```python
from build123d import *

# Parameters (mm, degrees)
F1_DEPTH = 5
F2_R     = 27
F2_R_2   = 25.5
F3_DEPTH = 5


# Not quite as in the source:
# - a feature names something its author has since deleted; it is built from what else it names


with BuildPart() as f1:
    # F0 (on Top) → F1 (new body)
    with BuildSketch(Plane.XY):
        with BuildLine():
            Line((26.83281573, 3), (23.8117617996, 3))
            ThreePointArc((23.8117617996, 3), (23.9528942217, 1.502949901), (24, 0))
            ThreePointArc((24, 0), (23.9528942217, -1.502949901), (23.8117617996, -3))
            Line((23.8117617996, -3), (26.83281573, -3))
            ThreePointArc((26.83281573, -3), (26.9581715321, -1.5023274094), (27, 0))
            ThreePointArc((27, 0), (26.9581715321, 1.5023274094), (26.83281573, 3))
        make_face()
        with BuildLine():
            ThreePointArc((3, 23.8117617996), (16.9705627485, 16.9705627485), (23.8117617996, 3))
            Line((23.8117617996, 3), (26.83281573, 3))
            ThreePointArc((26.83281573, 3), (19.091883092, 19.091883092), (3, 26.83281573))
            Line((3, 26.83281573), (3, 23.8117617996))
        make_face()
        with BuildLine():
            Line((26.83281573, -3), (23.8117617996, -3))
            ThreePointArc((23.8117617996, -3), (16.9705627485, -16.9705627485), (3, -23.8117617996))
            Line((3, -23.8117617996), (3, -26.83281573))
            ThreePointArc((3, -26.83281573), (19.091883092, -19.091883092), (26.83281573, -3))
        make_face()
        with BuildLine():
            ThreePointArc((-3, 23.8117617996), (0, 24), (3, 23.8117617996))
            Line((3, 23.8117617996), (3, 26.83281573))
            ThreePointArc((3, 26.83281573), (0, 27), (-3, 26.83281573))
            Line((-3, 26.83281573), (-3, 23.8117617996))
        make_face()
        with BuildLine():
            ThreePointArc((-23.8117617996, 3), (-16.9705627485, 16.9705627485), (-3, 23.8117617996))
            Line((-3, 23.8117617996), (-3, 26.83281573))
            ThreePointArc((-3, 26.83281573), (-19.091883092, 19.091883092), (-26.83281573, 3))
            Line((-26.83281573, 3), (-23.8117617996, 3))
        make_face()
        with BuildLine():
            Line((-3, -26.83281573), (-3, -23.8117617996))
            ThreePointArc((-3, -23.8117617996), (-16.9705627485, -16.9705627485), (-23.8117617996, -3))
            Line((-23.8117617996, -3), (-26.83281573, -3))
            ThreePointArc((-26.83281573, -3), (-19.091883092, -19.091883092), (-3, -26.83281573))
        make_face()
        with BuildLine():
            ThreePointArc((3, -23.8117617996), (0, -24), (-3, -23.8117617996))
            Line((-3, -23.8117617996), (-3, -26.83281573))
            ThreePointArc((-3, -26.83281573), (0, -27), (3, -26.83281573))
            Line((3, -26.83281573), (3, -23.8117617996))
        make_face()
        with BuildLine():
            ThreePointArc((-23.8117617996, -3), (-24, 0), (-23.8117617996, 3))
            Line((-23.8117617996, 3), (-26.83281573, 3))
            ThreePointArc((-26.83281573, 3), (-27, 0), (-26.83281573, -3))
            Line((-26.83281573, -3), (-23.8117617996, -3))
        make_face()
        with BuildLine():
            ThreePointArc((-6.7372564891, -3), (-7.2138024511, -1.5335185674), (-7.375, 0))
            ThreePointArc((-7.375, 0), (-7.2138024511, 1.5335185674), (-6.7372564891, 3))
            Line((-6.7372564891, 3), (-23.8117617996, 3))
            ThreePointArc((-23.8117617996, 3), (-24, 0), (-23.8117617996, -3))
            Line((-23.8117617996, -3), (-6.7372564891, -3))
        make_face()
        with BuildLine():
            ThreePointArc((-4.875, 0), (-3.4471455583, 3.4471455583), (0, 4.875))
            Line((0, 4.875), (0, 7.375))
            ThreePointArc((0, 7.375), (-1.5335185674, 7.2138024511), (-3, 6.7372564891))
            ThreePointArc((-3, 6.7372564891), (-5.2149125113, 5.2149125113), (-6.7372564891, 3))
            ThreePointArc((-6.7372564891, 3), (-7.2138024511, 1.5335185674), (-7.375, 0))
            Line((-7.375, 0), (-4.875, 0))
        make_face()
        with BuildLine():
            Line((0, -7.375), (0, -4.875))
            ThreePointArc((0, -4.875), (-3.4471455583, -3.4471455583), (-4.875, 0))
            Line((-4.875, 0), (-7.375, 0))
            ThreePointArc((-7.375, 0), (-7.2138024511, -1.5335185674), (-6.7372564891, -3))
            ThreePointArc((-6.7372564891, -3), (-5.2149125113, -5.2149125113), (-3, -6.7372564891))
            ThreePointArc((-3, -6.7372564891), (-1.5335185674, -7.2138024511), (0, -7.375))
        make_face()
        with BuildLine():
            Line((7.375, 0), (4.875, 0))
            ThreePointArc((4.875, 0), (3.4471455583, -3.4471455583), (0, -4.875))
            Line((0, -4.875), (0, -7.375))
            ThreePointArc((0, -7.375), (1.5335185674, -7.2138024511), (3, -6.7372564891))
            ThreePointArc((3, -6.7372564891), (5.2149125113, -5.2149125113), (6.7372564891, -3))
            ThreePointArc((6.7372564891, -3), (7.2138024511, -1.5335185674), (7.375, 0))
        make_face()
        with BuildLine():
            ThreePointArc((0, 4.875), (3.4471455583, 3.4471455583), (4.875, 0))
            Line((4.875, 0), (7.375, 0))
            ThreePointArc((7.375, 0), (7.2138024511, 1.5335185674), (6.7372564891, 3))
            ThreePointArc((6.7372564891, 3), (5.2149125113, 5.2149125113), (3, 6.7372564891))
            ThreePointArc((3, 6.7372564891), (1.5335185674, 7.2138024511), (0, 7.375))
            Line((0, 7.375), (0, 4.875))
        make_face()
        with BuildLine():
            ThreePointArc((-3, 6.7372564891), (-1.5335185674, 7.2138024511), (0, 7.375))
            ThreePointArc((0, 7.375), (1.5335185674, 7.2138024511), (3, 6.7372564891))
            Line((3, 6.7372564891), (3, 23.8117617996))
            ThreePointArc((3, 23.8117617996), (0, 24), (-3, 23.8117617996))
            Line((-3, 23.8117617996), (-3, 6.7372564891))
        make_face()
        with BuildLine():
            ThreePointArc((6.7372564891, 3), (7.2138024511, 1.5335185674), (7.375, 0))
            ThreePointArc((7.375, 0), (7.2138024511, -1.5335185674), (6.7372564891, -3))
            Line((6.7372564891, -3), (23.8117617996, -3))
            ThreePointArc((23.8117617996, -3), (23.9528942217, -1.502949901), (24, 0))
            ThreePointArc((24, 0), (23.9528942217, 1.502949901), (23.8117617996, 3))
            Line((23.8117617996, 3), (6.7372564891, 3))
        make_face()
        with BuildLine():
            ThreePointArc((3, -6.7372564891), (1.5335185674, -7.2138024511), (0, -7.375))
            ThreePointArc((0, -7.375), (-1.5335185674, -7.2138024511), (-3, -6.7372564891))
            Line((-3, -6.7372564891), (-3, -23.8117617996))
            ThreePointArc((-3, -23.8117617996), (0, -24), (3, -23.8117617996))
            Line((3, -23.8117617996), (3, -6.7372564891))
        make_face()
    extrude(amount=F1_DEPTH)

    # F2 (on face) → F3 (join)
    with BuildSketch(Plane.XY.offset(5)):
        Circle(F2_R)
        Circle(F2_R_2, mode=Mode.SUBTRACT)
    extrude(amount=F3_DEPTH)


solid = f1.part
```
Geometry check sheet. Reference: the model listing, model coordinates, mm. A direction names the side the tool comes from. Round coordinates to 2 decimals unless told otherwise and drop trailing zeros. Loops run counter-clockwise (first coordinate to the right, second up) from the corner with the lowest first, then second, coordinate; pieces in that order, holes last. Notation, with made-up numbers: (-24.75, 5.5) - (-17.75, 5.5) arc R17 ccw to (-17.75, 15.5) - close; hole circle Ø5 at (-27, -37). An arc over 180 degrees is marked (long way). Write each question's results on one line, items separated by ' | '. Start each with the question number.
Q1. Cross-section at C-C on z = 8. Enter the section's corners in (x, y), and give its area (3 significant figures).
Q2. Release check for a two-part mould opening along Y. For faces 1 (the flat face through (15, 3, 2)), 2 (the cylindrical face through (5.19, -5.24, 2.46)), 3 (the flat face through (24, -10, 10)) record: +Y half, -Y half, draft (parallel to the pull), parting line (faces both ways), or undercut.
Q3. Thickness scan on line 1 (X direction, y = 15, z = 2) (3 decimals); line 2 (Y direction, x = 0, z = 6.1); line 3 (Y direction, x = -6.5, z = 3.75). Record the ranges inside material, lowest first. Write a range as [from, to].
Q4. Cross-section at B-B on x = 16. Enter the section's corners in (y, z).
Q5. Access from +Z, -Z, +X, -X, +Y, -Y to the whole of each face (thin tool, end or side, straight path). Record for faces 4 (the flat face through (6, 0, 0)), 5 (the cylindrical face through (-5.5, -24.9, 7.5)), 6 (the cylindrical face through (16.81, 17.13, 2.46)).
Q6. Cross-section at A-A on y = -21. Enter the section's corners in (x, z), and give its area (3 significant figures).
Q7. Gauge pin test, flat ends, axial feed: P1, Ø4, axis at y = 6, z = 7.5, coming from the -X side; P2, Ø1.5, axis at x = -15, z = 3, coming from the -Y side; P3, Ø5.5, axis at x = 18, z = 1.5, coming from the +Y side. Record the tip position at first contact, or that the pin passes through.
Answers below:
1) outline: circle Ø54 at (0, 0); hole circle Ø51 at (0, 0) | area: 247 mm²
2) face 1: undercut | face 2: undercut | face 3: draft
3) line 1: x = [-22.45, -18.735], [-3, 3], [18.735, 22.45] | line 2: y = [-27, -25.5], [25.5, 27] | line 3: y = [-26.21, -23.1], [-3.48, 3.48], [23.1, 26.21]
4) outline: (-21.75, 0) - (-17.89, 0) - (-17.89, 5) - (-19.86, 5) - (-19.86, 10) - (-21.75, 10) - close; (-3, 0) - (3, 0) - (3, 5) - (-3, 5) - close; (17.89, 0) - (21.75, 0) - (21.75, 10) - (19.86, 10) - (19.86, 5) - (17.89, 5) - close
5) face 4: -Z, +X, -X, +Y, -Y | face 5: +Z | face 6: +Z, -Z
6) outline: (-16.97, 0) - (-11.62, 0) - (-11.62, 5) - (-14.47, 5) - (-14.47, 10) - (-16.97, 10) - close; (-3, 0) - (3, 0) - (3, 5) - (-3, 5) - close; (11.62, 0) - (16.97, 0) - (16.97, 10) - (14.47, 10) - (14.47, 5) - (11.62, 5) - close | area: 109 mm²
7) P1: stops at x = -26.7 | P2: stops at y = -22.93 | P3: stops at y = 22.28
